Work out the finished part from the listing and answer in its coordinate system (mm). Face numbers are marked on the shaded views. A direction names the side the tool comes from. Round coordinates to 2 decimals unless told otherwise and drop trailing zeros.
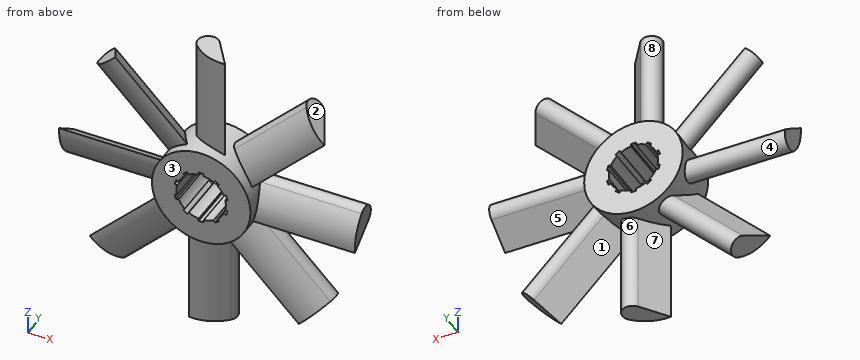
from build123d import *

# Parameters (mm, degrees)
F0_R            = 12.7
F0_R_2          = 6.35
F1_DEPTH        = 6.35
F4_DEPTH        = 25.4
F7_DEPTH        = 30.48
F7_COPIES_COUNT = 8


# Not quite as in the source:
# - a pattern or mirror of a feature is missing from the dataset's text; its kind, count and spacing are read off the source's solid


with BuildPart() as f1:
    # F0 (on Front) → F1 (new body, symmetric)
    with BuildSketch(Plane.XZ):
        Circle(F0_R)
        Circle(F0_R_2, mode=Mode.SUBTRACT)
    extrude(amount=F1_DEPTH, both=True)

    # F3 (on offset) → F4 (cut)
    with BuildSketch(Plane.XZ.offset(6.35)):
        with BuildLine():
            Line((-3.2000014887, 5.4847507211), (-3.5919541958, 6.0242273409))
            Line((-3.5919541958, 6.0242273409), (-4.6194057787, 5.2777400705))
            Line((-4.6194057787, 5.2777400705), (-4.2274530715, 4.7382634507))
            ThreePointArc((-4.2274530715, 4.7382634507), (-3.7324363521, 5.1372579143), (-3.2000014887, 5.4847507211))
        make_face()
        with BuildLine():
            ThreePointArc((-0.635, 6.3181702256), (0, 6.35), (0.635, 6.3181702256))
            Line((0.635, 6.3181702256), (0.635, 6.985))
            Line((0.635, 6.985), (-0.635, 6.985))
            Line((-0.635, 6.985), (-0.635, 6.3181702256))
        make_face()
        with BuildLine():
            Line((4.2274530715, 4.7382634507), (4.6194057787, 5.2777400705))
            Line((4.6194057787, 5.2777400705), (3.5919541958, 6.0242273409))
            Line((3.5919541958, 6.0242273409), (3.2000014887, 5.4847507211))
            ThreePointArc((3.2000014887, 5.4847507211), (3.7324363521, 5.1372579143), (4.2274530715, 4.7382634507))
        make_face()
        with BuildLine():
            Line((6.2051627556, 1.3485010852), (6.8393555577, 1.5545628179))
            Line((6.8393555577, 1.5545628179), (6.4469039749, 2.7624045936))
            Line((6.4469039749, 2.7624045936), (5.8127111727, 2.5563428609))
            ThreePointArc((5.8127111727, 2.5563428609), (6.0392088785, 1.9622579143), (6.2051627556, 1.3485010852))
        make_face()
        with BuildLine():
            Line((5.8127111727, -2.5563428609), (6.4469039749, -2.7624045936))
            Line((6.4469039749, -2.7624045936), (6.8393555577, -1.5545628179))
            Line((6.8393555577, -1.5545628179), (6.2051627556, -1.3485010852))
            ThreePointArc((6.2051627556, -1.3485010852), (6.0392088785, -1.9622579143), (5.8127111727, -2.5563428609))
        make_face()
        with BuildLine():
            Line((-6.2051627556, -1.3485010852), (-6.8393555577, -1.5545628179))
            Line((-6.8393555577, -1.5545628179), (-6.4469039749, -2.7624045936))
            Line((-6.4469039749, -2.7624045936), (-5.8127111727, -2.5563428609))
            ThreePointArc((-5.8127111727, -2.5563428609), (-6.0392088785, -1.9622579143), (-6.2051627556, -1.3485010852))
        make_face()
        with BuildLine():
            Line((-5.8127111727, 2.5563428609), (-6.4469039749, 2.7624045936))
            Line((-6.4469039749, 2.7624045936), (-6.8393555577, 1.5545628179))
            Line((-6.8393555577, 1.5545628179), (-6.2051627556, 1.3485010852))
            ThreePointArc((-6.2051627556, 1.3485010852), (-6.0392088785, 1.9622579143), (-5.8127111727, 2.5563428609))
        make_face()
        with BuildLine():
            Line((-4.2274530715, -4.7382634507), (-4.6194057787, -5.2777400705))
            Line((-4.6194057787, -5.2777400705), (-3.5919541958, -6.0242273409))
            Line((-3.5919541958, -6.0242273409), (-3.2000014887, -5.4847507211))
            ThreePointArc((-3.2000014887, -5.4847507211), (-3.7324363521, -5.1372579143), (-4.2274530715, -4.7382634507))
        make_face()
        with BuildLine():
            Line((-0.635, -6.3181702256), (-0.635, -6.985))
            Line((-0.635, -6.985), (0.635, -6.985))
            Line((0.635, -6.985), (0.635, -6.3181702256))
            ThreePointArc((0.635, -6.3181702256), (0, -6.35), (-0.635, -6.3181702256))
        make_face()
        with BuildLine():
            Line((3.2000014887, -5.4847507211), (3.5919541958, -6.0242273409))
            Line((3.5919541958, -6.0242273409), (4.6194057787, -5.2777400705))
            Line((4.6194057787, -5.2777400705), (4.2274530715, -4.7382634507))
            ThreePointArc((4.2274530715, -4.7382634507), (3.7324363521, -5.1372579143), (3.2000014887, -5.4847507211))
        make_face()
    extrude(amount=-F4_DEPTH, mode=Mode.SUBTRACT)

    # F6 (on offset) → F7 (join)
    with BuildSketch(Plane.YZ.offset(38.1)):
        with BuildLine():
            ThreePointArc((0, 4.386866935), (-2.7218067049, 0.2512213266), (-3.4407728063, -4.64723599))
            Line((-3.4407728063, -4.64723599), (3.4407728063, 0.260369055))
            ThreePointArc((3.4407728063, 0.260369055), (3.9456637131, 4.1791075354), (0, 4.386866935))
        make_face()
    f7 = extrude(amount=-F7_DEPTH)

    # F7_copies: F7 ×8 about axis
    f7_copies_axis = Axis((0, 0, 0), (0, 1, 0))
    for i in range(1, F7_COPIES_COUNT):
        add(f7.rotate(f7_copies_axis, i * 360 / F7_COPIES_COUNT))


solid = f1.part
Q1. Find the intervals of material crossed by L1, parallel to X at y = 1.25, z = 14; L2, parallel to Z at x = -13.5, y = 3; L3, parallel to X at y = 1.5, z = -17.5, in increasing order.
Q2. A tool of negligible diameter and unlimited length cuts with its end or side. For the marked faces 4, 5, 6, 7 and 8, from which of +Z, -Z, +X, -X, +Y, -Y can it reach the whole face along a straight path? Write none if from no direction.
Q3. Find section B-B (z = 14.5). Count the separate pieces of the cut face and the enclosed holes in it, plus the area to 3 significant figures.
Q4. Given pin 1 (1 mm diameter, centred on x = 12, z = 15.5, fed in from -Y); pin 2 (0.7 mm diameter, centred on y = 2, z = 7, fed in from +X); pin 3 (4 mm diameter, centred on x = -25.5, y = -4, fed in from +Z); pin 4 (1.5 mm diameter, centred on y = -5, z = 20.5, fed in from -X), each flat-ended and moving along its own axis, determine where each tip first touches the part or whether it passes through.
Q5. The mould has two halves that part along X. Classify the marked faces 1, 2 and 3: +X half, -X half, draft (parallel to the pull), parting line (faces both ways), or undercut.
Report:
1. L1: x = -21.18 to -12.16, -5.07 to 1.3, 6.82 to 15.84
1. L2: z = -20.43 to -13.42, -4.9 to 0.05, 6.57 to 13.58
1. L3: x = -19.09 to -10.26, -1.12 to 5.12, 15.91 to 24.74
2. face 4: -X
2. face 5: +X, +Y
2. face 6: -Z
2. face 7: -Z, +Y
2. face 8: +Z
3. separate pieces: 3
3. enclosed holes: 0
3. area: 161 mm2
4. pin 1: stops at y = -1.89
4. pin 2: stops at x = 10.82
4. pin 3: stops at z = 30.23
4. pin 4: passes through
5. face 1: undercut
5. face 2: +X half
5. face 3: draft
